```python
from build123d import *

# Parameters (mm, degrees)
EXTRUDE_1_DEPTH          = 6
EXTRUDE_START            = -3.991967
EXTRUDE_2_DEPTH          = 3.991967
PATTERN_CIRCULAR_1_COUNT = 5
PATTERN_CIRCULAR_1_ANGLE = 180
SKETCH_4_R               = 3
CUT_EXTRUDE_1_DEPTH      = 7.0000001


with BuildPart() as part:
    # Sketch 1 → Extrude 1 (new body)
    with BuildSketch(Plane.XY):
        with BuildLine():
            Line((-4.5, 0), (-4.5, -18.2))
            Line((-4.5, -18.2), (-3, -18.2))
            Line((-3, -18.2), (-3, -14.6))
            ThreePointArc((-3, -14.6), (-1.968245837, -12.85), (-3, -11.1))
            Line((-3, -11.1), (-3, -10))
            Line((-3, -10), (3, -10))
            Line((3, -10), (3, -11.1))
            ThreePointArc((3, -11.1), (1.968245837, -12.85), (3, -14.6))
            Line((3, -14.6), (3, -18.2))
            Line((3, -18.2), (4.5, -18.2))
            Line((4.5, -18.2), (4.5, 0))
            ThreePointArc((4.5, 0), (0, 4.5), (-4.5, 0))
        make_face()
    extrude_1 = extrude(amount=EXTRUDE_1_DEPTH)

    # Sketch 3 → Extrude 2 (add)
    with BuildSketch(Plane.XZ.offset(18.2).offset(EXTRUDE_START)):
        with BuildLine():
            Line((-3, 6), (-3, 0))
            Line((-3, 0), (-2.5, 1))
            Line((-2.5, 1), (-2.5, 1.5))
            ThreePointArc((-2.5, 1.5), (-2.757359313, 3), (-2.5, 4.5))
            Line((-2.5, 4.5), (-2.5, 5))
            Line((-2.5, 5), (-3, 6))
        make_face()
        with BuildLine():
            Line((3, 0), (2.5, 1))
            Line((2.5, 1), (2.5, 1.5))
            ThreePointArc((2.5, 1.5), (2.757359313, 3), (2.5, 4.5))
            Line((2.5, 4.5), (2.5, 5))
            Line((2.5, 5), (3, 6))
            Line((3, 6), (3, 0))
        make_face()
    extrude_2 = extrude(amount=EXTRUDE_2_DEPTH)

    # Pattern Circular 1: Extrude 1, Extrude 2 ×5 about axis
    pattern_circular_1_axis = Axis((0, 0, 0), (0, 0, 1))
    for i in range(1, PATTERN_CIRCULAR_1_COUNT):
        add(extrude_1.rotate(pattern_circular_1_axis, i * PATTERN_CIRCULAR_1_ANGLE / (PATTERN_CIRCULAR_1_COUNT - 1)))
        add(extrude_2.rotate(pattern_circular_1_axis, i * PATTERN_CIRCULAR_1_ANGLE / (PATTERN_CIRCULAR_1_COUNT - 1)))

    # Sketch 4 → Cut-Extrude 1 (cut, through all)
    with BuildSketch(Plane(origin=(0, 0, 0), x_dir=(-1, 0, 0), z_dir=(0, 0, -1))):
        Circle(SKETCH_4_R)
        with BuildLine():
            Line((3, -8.75), (3, -3.354101966))
            ThreePointArc((3, -3.354101966), (1.038095674, -4.378625055), (-1.174936357, -4.343906601))
            Line((-1.174936357, -4.343906601), (-3, -8.75))
            Line((-3, -8.75), (3, -8.75))
        make_face()
        with BuildLine():
            Line((-4.065863992, -8.308504679), (-8.308504679, -4.065863992))
            Line((-8.308504679, -4.065863992), (-3.90241128, -2.240800349))
            ThreePointArc((-3.90241128, -2.240800349), (-3.181980515, -3.181980515), (-2.240800349, -3.90241128))
            Line((-2.240800349, -3.90241128), (-4.065863992, -8.308504679))
        make_face()
        with BuildLine():
            Line((3, 8.75), (3, 3.354101966))
            ThreePointArc((3, 3.354101966), (1.038095674, 4.378625055), (-1.174936357, 4.343906601))
            Line((-1.174936357, 4.343906601), (-3, 8.75))
            Line((-3, 8.75), (3, 8.75))
        make_face()
        with BuildLine():
            Line((-8.75, 3), (-4.343906601, 1.174936357))
            ThreePointArc((-4.343906601, 1.174936357), (-4.5, 0), (-4.343906601, -1.174936357))
            Line((-4.343906601, -1.174936357), (-8.75, -3))
            Line((-8.75, -3), (-8.75, 3))
        make_face()
        with BuildLine():
            Line((-4.065863992, 8.308504679), (-2.240800349, 3.90241128))
            ThreePointArc((-2.240800349, 3.90241128), (-3.181980515, 3.181980515), (-3.90241128, 2.240800349))
            Line((-3.90241128, 2.240800349), (-8.308504679, 4.065863992))
            Line((-8.308504679, 4.065863992), (-4.065863992, 8.308504679))
        make_face()
    extrude(amount=-CUT_EXTRUDE_1_DEPTH, mode=Mode.SUBTRACT)


solid = part.part
```
Here's how the part is built. I have some questions about the finished solid (model axes, mm). A direction names the side the tool comes from. Coordinates: 2 decimals unless noted, no trailing zeros. Write each loop counter-clockwise with the first axis right and the second up, starting at its lowest first coordinate (ties: lowest second). Pieces come first, ordered by that corner, then holes. Notation, with made-up numbers: (8.25, 68.25) -> (50.25, 68.25) arc R31 cw to (50.25, 98.25) -> close; hole circle Ø9 at (52, -27.5). An arc over 180 degrees is marked (long way). Use a Markdown table: item, result. Add a question column.
(1) For faces 1 (the flat face through (-2.746, 16.176, 5.493)), 2 (the flat face through (13.385, -9.491, 0.493)), 3 (the cylindrical face through (2.757, -16.176, 2.979)), 4 (the flat face through (6.516, -2.075, 2.958)), 5 (the flat face through (13.421, 7.057, 2.958)), which set-ups out of +Z, -Z, +X, -X, +Y, -Y let a thin tool reach every point of the face, with its end or its side?
(2) If we section it at A-A, the plane x = 0: Write out the boundary of the cut face in (y, z).
(3) I'm going to push flat-ended pins straight in: P1, Ø1.6, axis at y = 6, z = 2.5, coming from the +X side; P2, Ø0.5, axis at x = 10.5, z = 2.5, coming from the +Y side; P3, Ø1.8, axis at y = -1.5, z = 3.5, coming from the +X side. Where does each tip first touch, or does it pass through?
(4) If we section it at B-B, the plane y = 0: Write out the boundary of the cut face in (x, z), and give its area (3 significant figures).
(5) We'd pull the mould along Y, two halves only. Please class faces 6 (the flat face through (9.491, -13.385, 0.493)), 7 (the flat face through (-4.5, 0, 3)), 8 (the flat face through (7.13, 13.494, 2.958)), 9 (the flat face through (3.166, 6.136, 2.958)): +Y half, -Y half, draft (parallel to the pull), parting line (faces both ways), or undercut.
(6) If we section it at D-D, the plane y = -7: Write out the boundary of the cut face in (x, z), and give its area (3 significant figures).
(7) Please list where these lines run through material, in increasing order: line 1 (Y direction, x = 0, z = 4.55); line 2 (X direction, y = 5.5, z = 2.75); line 3 (Y direction, x = 10.75, z = 5).
(8) If we section it at C-C, the plane x = 6.5: Write out the boundary of the cut face in (y, z).
Outcome:
| question | item | result |
|---|---|---|
| 1 | face 1 | +Z, +Y |
| 1 | face 2 | -Z, -Y |
| 1 | face 3 | -Y |
| 1 | face 4 | +Z, -Z |
| 1 | face 5 | +Z, -Z, +X |
| 2 | outline | (-10, 0) -> (-8.75, 0) -> (-8.75, 6) -> (-10, 6) -> close; (-4.5, 0) -> (-3, 0) -> (-3, 6) -> (-4.5, 6) -> close; (3, 0) -> (4.5, 0) -> (4.5, 6) -> (3, 6) -> close; (8.75, 0) -> (10, 0) -> (10, 6) -> (8.75, 6) -> close |
| 3 | P1 | stops at x = 13.16 |
| 3 | P2 | stops at y = 15.49 |
| 3 | P3 | stops at x = 14.09 |
| 4 | outline | (-4.5, 0) -> (-3, 0) -> (-3, 6) -> (-4.5, 6) -> close; (3, 0) -> (4.5, 0) -> (4.5, 6) -> (3, 6) -> close; (8.75, 0) -> (10, 0) -> (10, 6) -> (8.75, 6) -> close |
| 4 | area | 25.5 mm^2 |
| 5 | face 6 | undercut |
| 5 | face 7 | draft |
| 5 | face 8 | +Y half |
| 5 | face 9 | undercut |
| 6 | outline | (-4.5, 0) -> (-3, 0) -> (-3, 6) -> (-4.5, 6) -> close; (2.28, 0) -> (3.52, 0) -> (3.52, 6) -> (2.28, 6) -> close; (5.37, 0) -> (7.14, 0) -> (7.14, 6) -> (5.37, 6) -> close; (10.03, 0) -> (13.36, 0) -> (13.36, 6) -> (10.03, 6) -> close |
| 6 | area | 47.1 mm^2 |
| 7 | line 1 | y = -10 to -8.75, -4.5 to -3, 3 to 4.5, 8.75 to 10 |
| 7 | line 2 | x = -4.5 to -3, 1.65 to 2.9, 6.87 to 8.64, 9.74 to 11.86 |
| 7 | line 3 | y = -14.99 to -14.29, -7.92 to -3, 3 to 7.92, 14.29 to 14.99 |
| 8 | outline | (-12.86, 0) -> (-9.9, 0) -> (-9.9, 6) -> (-12.86, 6) -> close; (-7.64, 0) -> (-5.87, 0) -> (-5.87, 6) -> (-7.64, 6) -> close; (-3.32, 0) -> (-2.07, 0) -> (-2.07, 6) -> (-3.32, 6) -> close; (2.07, 0) -> (3.32, 0) -> (3.32, 6) -> (2.07, 6) -> close; (5.87, 0) -> (7.64, 0) -> (7.64, 6) -> (5.87, 6) -> close; (9.9, 0) -> (12.86, 0) -> (12.86, 6) -> (9.9, 6) -> close |
